Input: part model. Units: mm. Frame: model coordinates. Round coordinates to 2 decimals unless told otherwise and drop trailing zeros. Order: outer loops, then holes, each group sorted by start corner. A loop starts at its lowest first (then second) coordinate and runs counter-clockwise, first axis right, second up. Notation, with made-up numbers: (18.5, 80.5) -> (26.5, 80.5) arc R28 cw to (26.5, 110.5) -> close; hole circle Ø11 at (-34.5, -10.5). An arc over 180 degrees is marked (long way). Answer as CSV lines item,"result". Start each with the question number.
1) Section query B-B, the plane z = -13.5. Output: boundary loops of the cut face in (x, y), and give its area (3 significant figures).
2) Section query A-A, the plane y = 0.6. Output: boundary loops of the cut face in (x, z), and give its area (3 significant figures).
3) Section query D-D, the plane x = -5. Output: boundary loops of the cut face in (y, z).
4) Section query C-C, the plane x = 0. Output: boundary loops of the cut face in (y, z), and give its area (3 significant figures).
5) Line query: L1, parallel to X at y = 2.25, z = 5.5; L2, parallel to X at y = 1.4, z = -10; L3, parallel to Z at x = -8, y = 2.3. Output: solid intervals per line, ascending.
6) First-contact query: P1, Ø1.8, axis at x = 15.5, z = -25.5, coming from the +Y side. Flat tip, straight axial feed; report the tip coordinate or a pass-through.
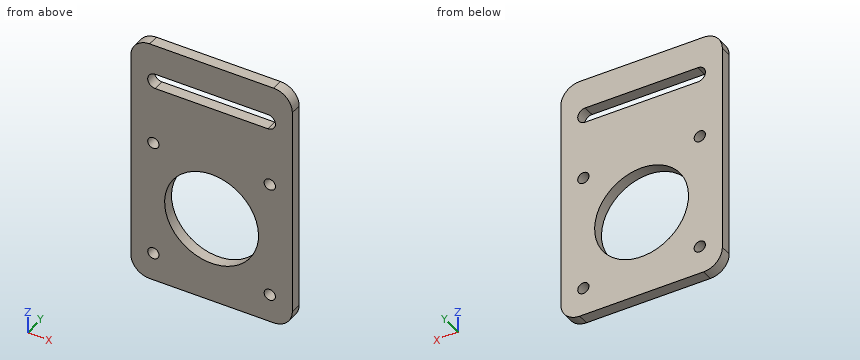
```python
from build123d import *

# Parameters (mm, degrees)
SKETCH1_W           = 43
SKETCH1_H           = 66
BOSS_EXTRUDE1_DEPTH = 3
SKETCH2_R           = 1.5
SKETCH2_R_2         = 12.5
CUT_EXTRUDE1_DEPTH  = 40.5
FILLET1_R           = 5


with BuildPart() as part:
    # Sketch1 → Boss-Extrude1 (new body)
    with BuildSketch(Plane(origin=(0, 0, 0), x_dir=(1, 0, 0), z_dir=(0, 1, 0))):
        Rectangle(SKETCH1_W, SKETCH1_H)
    extrude(amount=BOSS_EXTRUDE1_DEPTH)

    # Sketch2 → Cut-Extrude1 (cut, through all)
    with BuildSketch(Plane(origin=(0, 3, 0), x_dir=(1, 0, 0), z_dir=(0, 1, 0))):
        with Locations(Location((15.5, 25.5, 0), (0, 0, 270))):
            Circle(SKETCH2_R)
        with Locations(Location((-15.5, 25.5, 0), (0, 0, 270))):
            Circle(SKETCH2_R)
        with Locations(Location((-15.5, -5.5, 0), (0, 0, 270))):
            Circle(SKETCH2_R)
        with Locations(Location((15.5, -5.5, 0), (0, 0, 270))):
            Circle(SKETCH2_R)
        with Locations(Location((0, 10, 0), (0, 0, 270))):
            Circle(SKETCH2_R_2)
        with BuildLine():
            Line((-15, -21), (15, -21))
            ThreePointArc((15, -21), (17, -23), (15, -25))
            Line((15, -25), (-15, -25))
            ThreePointArc((-15, -25), (-17, -23), (-15, -21))
        make_face()
    extrude(amount=-CUT_EXTRUDE1_DEPTH, mode=Mode.SUBTRACT)

    # Fillet1
    fillet1_edges = [part.edges().sort_by_distance(p)[0] for p in [
        (-21.5, 1.5, -33),
        (21.5, 1.5, -33),
        (21.5, 1.5, 33),
        (-21.5, 1.5, 33),
    ]]
    fillet(fillet1_edges, radius=FILLET1_R)


solid = part.part
```
Findings:
1,outline,"(-21.5, 0) -> (-12, 0) -> (-12, 3) -> (-21.5, 3) -> close; (12, 0) -> (21.5, 0) -> (21.5, 3) -> (12, 3) -> close"
1,area,"57.0 mm^2"
2,outline,"(-21.5, -28) arc R5 ccw to (-16.5, -33) -> (16.5, -33) arc R5 ccw to (21.5, -28) -> (21.5, 28) arc R5 ccw to (16.5, 33) -> (-16.5, 33) arc R5 ccw to (-21.5, 28) -> close; hole circle Ø3 at (-15.5, -25.5); hole circle Ø3 at (-15.5, 5.5); hole (-15, 21) -> (15, 21) arc R2 ccw to (15, 25) -> (-15, 25) arc R2 ccw to start; hole circle Ø25 at (0, -10); hole circle Ø3 at (15.5, -25.5); hole circle Ø3 at (15.5, 5.5)"
2,area,"2,160 mm^2"
3,outline,"(0, -33) -> (3, -33) -> (3, -21.46) -> (0, -21.46) -> close; (0, 1.46) -> (3, 1.46) -> (3, 21) -> (0, 21) -> close; (0, 25) -> (3, 25) -> (3, 33) -> (0, 33) -> close"
4,outline,"(0, -33) -> (3, -33) -> (3, -22.5) -> (0, -22.5) -> close; (0, 2.5) -> (3, 2.5) -> (3, 21) -> (0, 21) -> close; (0, 25) -> (3, 25) -> (3, 33) -> (0, 33) -> close"
4,area,"111 mm^2"
5,L1,"x = -21.5 to -17, -14 to 14, 17 to 21.5"
5,L2,"x = -21.5 to -12.5, 12.5 to 21.5"
5,L3,"z = -33 to -19.6, -0.4 to 21, 25 to 33"
6,P1,"passes through"
